Design review of the part shown in the three views and the two pictorial views. Dimensions are in mm from the part's minimum x, y and z. Coordinates: 2 decimals unless noted, no trailing zeros. Loops run counter-clockwise (first coordinate to the right, second up) from the corner with the lowest first, then second, coordinate; pieces in that order, holes last.
Q1. For P1, Ø4, axis at y = 3, z = 12, coming from the +X side, flat-tipped, find the tip position at first contact; note if it passes through.
Q2. Add section A-A on x = 4. Give the boundary of the cut face in (y, z).
Q3. Wall thickness on probe 1 along Y at (x, z) = (6.75, 5.5) (1 decimal); probe 2 along Y at (x, z) = (7, 4.5) (1 decimal); probe 3 along X at (y, z) = (4.25, 9.25): over which ranges is each line inside the solid? List them lowest first.
Q4. Add section D-D on z = 2.25. Give the boundary of the cut face in (x, y).
Q5. Add section C-C on z = 11.5. Give the boundary of the cut face in (x, y).
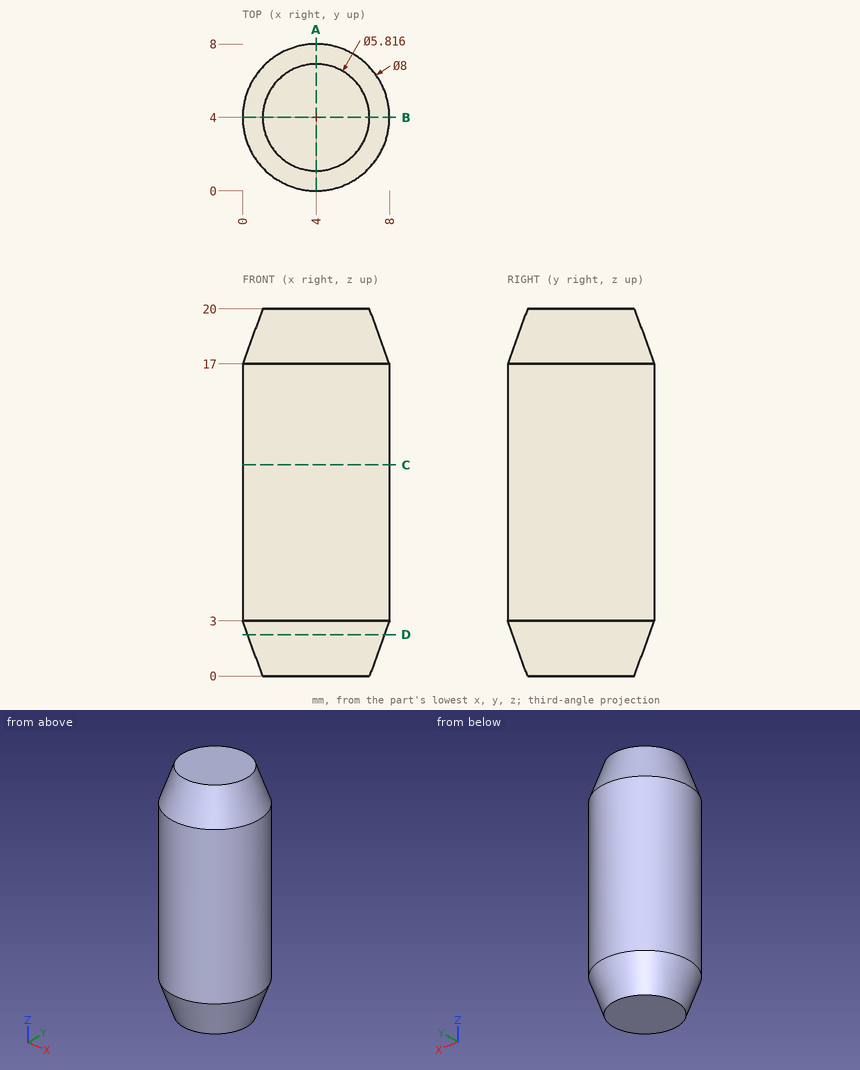
Entries:
1. P1: stops at x = 8
2. outline: (0, 3) - (1.09, 0) - (6.91, 0) - (8, 3) - (8, 17) - (6.91, 20) - (1.09, 20) - (0, 17) - close
3. probe 1: y = 1.1 to 6.9
3. probe 2: y = 1.4 to 6.6
3. probe 3: x = 0.01 to 7.99
4. outline: circle Ø7.45 at (4, 4)
5. outline: circle Ø8 at (4, 4)
